The model under review builds one solid part; all positions refer to its coordinate system, in mm. Face numbers are marked on the shaded views. A direction names the side the tool comes from. Give positions to 0.01 mm unless a question says otherwise; leave off trailing zeros. Loops run counter-clockwise (first coordinate to the right, second up) from the corner with the lowest first, then second, coordinate; pieces in that order, holes last. Notation, with made-up numbers: M -2.75,36.5 L 5.25,36.5 A15 cw 5.25,62.5 Z; hole C 23.5,86 d4. An arc over 180 degrees is marked long. Return JSON: item names as keys, results as strings.
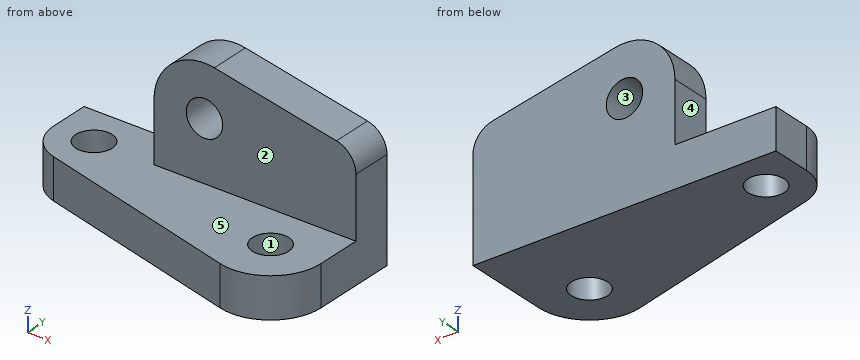
```python
from build123d import *

# Parameters (mm, degrees)
F1_DEPTH = 20
F3_DEPTH = 20
F4_R     = 20
F5_R     = 25
F6_R     = 25
F7_R     = 12
F10_D    = 18
F11_D    = 18
F13_D    = 18


with BuildPart() as f1:
    # F0 (on Top) → F1 (new body)
    with BuildSketch(Plane.XY):
        Polygon((51.892916, 64.117395), (-98.107084, 64.117395), (-98.107084, 29.117395), (51.892916, -10.882605), align=None)
    extrude(amount=F1_DEPTH)

    # F2 (on face) → F3 (join)
    with BuildSketch(Plane(origin=(0, 64.117395, 0), x_dir=(-1, 0, 0), z_dir=(0, 1, 0))):
        Polygon((-51.892916, 60), (-51.892916, 20), (48.107084, 20), (48.107084, 80), align=None)
    extrude(amount=-F3_DEPTH)

    # F4
    f4_edges = [f1.edges().sort_by_distance(p)[0] for p in [
        (-98.107084, 29.117395, 10),
    ]]
    fillet(f4_edges, radius=F4_R)

    # F5
    f5_edges = [f1.edges().sort_by_distance(p)[0] for p in [
        (51.892916, -10.882605, 10),
    ]]
    fillet(f5_edges, radius=F5_R)

    # F6
    f6_edges = [f1.edges().sort_by_distance(p)[0] for p in [
        (-48.107084, 54.117395, 80),
    ]]
    fillet(f6_edges, radius=F6_R)

    # F7
    f7_edges = [f1.edges().sort_by_distance(p)[0] for p in [
        (51.892916, 54.117395, 60),
    ]]
    fillet(f7_edges, radius=F7_R)

    # F10 (through all)
    with Locations(Plane.XZ.offset(-44.117395)):
        with Locations((-23.107084, 49.504902)):
            Hole(F10_D / 2)

    # F11 (through all)
    with Locations(Plane.XY.offset(20)):
        with Locations((-78.107084, 44.482961)):
            Hole(F11_D / 2)

    # F13 (through all)
    with Locations(Plane.XY.offset(20)):
        with Locations((26.892916, 21.657686)):
            Hole(F13_D / 2)


solid = f1.part
```
1) Consider section A-A on y = 16. Write out the cut boundary in (x, z).
From the geometry:
{"outline": "M -48.92,0 L 19.89,0 L 19.89,20 L -48.92,20 Z; M 33.89,0 L 51.24,0 L 51.24,20 L 33.89,20 Z"}
2) Consider section B-B on x = -26.5. Write out the cut boundary in (y, z), then the cut area to 3 significant figures.
From the geometry:
{"outline": "M 10.02,0 L 64.12,0 L 64.12,41.17 L 44.12,41.17 L 44.12,20 L 10.02,20 Z; M 44.12,57.84 L 64.12,57.84 L 64.12,74.27 L 44.12,74.27 Z", "area": "1,830 mm²"}
3) Consider section C-C on z = 56.5. Write out the cut boundary in (x, y), then the cut area to 3 significant figures.
From the geometry:
{"outline": "M -47.11,44.12 L -28.77,44.12 L -28.77,64.12 L -47.11,64.12 Z; M -17.44,44.12 L 50.08,44.12 L 50.08,64.12 L -17.44,64.12 Z", "area": "1,720 mm²"}
4) Wall thickness on L1, parallel to Z at x = -1, y = 42; L2, parallel to Y at x = 36, z = 58.5; L3, parallel to Y at x = -80.5, z = 9.5: over which ranges is each line inside the solid? List them lowest first. Write a range as from..to.
From the geometry:
{"L1": "0..20", "L2": "44.12..64.12", "L3": "24.42..35.81, 53.16..64.12"}
5) Insertion check: pin 1 (1 mm diameter, centred on x = 15, z = 13.5, fed in from -Y); pin 2 (16 mm diameter, centred on y = 58.5, z = 29, fed in from -X); pin 3 (12 mm diameter, centred on x = 12, y = 18, fed in from +Z). Each pin has a flat end and moves straight along its axis. Give the tip position at first contact, or say it passes through.
From the geometry:
{"pin 1": "y = -1.18", "pin 2": "x = -48.11", "pin 3": "z = 20"}
6) The part is to be moulded in two halves that separate along X. For the marked faces 3, 4 and 5, say which applies: released by +X, released by -X, zero draft, split by the parting line, or undercut.
From the geometry:
{"face 3": "undercut", "face 4": "released by -X", "face 5": "zero draft"}
7) Tool access review of the marked faces 1 and 2: name each direction out of +Z, -Z, +X, -X, +Y, -Y from which nothing blocks a thin tool from reaching the whole face with its end or side.
From the geometry:
{"face 1": "+Z, -Z", "face 2": "+Z, +X, -X, -Y"}
8) Consider section D-D on x = 26. Write out the cut boundary in (y, z).
From the geometry:
{"outline": "M -3.33,0 L 12.7,0 L 12.7,20 L -3.33,20 Z; M 30.61,0 L 64.12,0 L 64.12,65.18 L 44.12,65.18 L 44.12,20 L 30.61,20 Z"}
